```python
from build123d import *

# Parameters (mm, degrees)
EXTRUDE_268_DEPTH      = 3
SKETCH_2_W             = 50
SKETCH_2_H             = 30
CUT_EXTRUDE_486_DEPTH  = 121.867696263
SKETCH_3_R             = 2.5
CUT_EXTRUDE_744_DEPTH  = 121.867696263
SKETCH_4_R             = 2.6
CUT_EXTRUDE_1056_DEPTH = 121.867696263


with BuildPart() as part:
    # 草图1 → Extrude 268 (new body)
    with BuildSketch(Plane(origin=(0, 0, 0), x_dir=(1, 0, 0), z_dir=(0, 1, 0))):
        with BuildLine():
            Line((-100, 50), (100, 50))
            ThreePointArc((100, 50), (107.071067812, 47.071067812), (110, 40))
            Line((110, 40), (110, -40))
            ThreePointArc((110, -40), (107.071067812, -47.071067812), (100, -50))
            Line((100, -50), (-100, -50))
            ThreePointArc((-100, -50), (-107.071067812, -47.071067812), (-110, -40))
            Line((-110, -40), (-110, 40))
            ThreePointArc((-110, 40), (-107.071067812, 47.071067812), (-100, 50))
        make_face()
    extrude(amount=EXTRUDE_268_DEPTH)

    # 草图2 → Cut-Extrude 486 (cut, through all)
    with BuildSketch(Plane(origin=(0, 3, 0), x_dir=(1, 0, 0), z_dir=(0, 1, 0))):
        with Locations((0, 35)):
            Rectangle(SKETCH_2_W, SKETCH_2_H)
    extrude(amount=-CUT_EXTRUDE_486_DEPTH, mode=Mode.SUBTRACT)

    # 草图3 → Cut-Extrude 744 (cut, through all)
    with BuildSketch(Plane(origin=(0, 3, 0), x_dir=(1, 0, 0), z_dir=(0, 1, 0))):
        with Locations(Location((10, 8, 0), (0, 0, 270))):
            Circle(SKETCH_3_R)
        with Locations(Location((10, -12, 0), (0, 0, 270))):
            Circle(SKETCH_3_R)
        with Locations(Location((10, -32, 0), (0, 0, 270))):
            Circle(SKETCH_3_R)
        with Locations(Location((-10, -32, 0), (0, 0, 270))):
            Circle(SKETCH_3_R)
        with Locations(Location((-10, -12, 0), (0, 0, 270))):
            Circle(SKETCH_3_R)
        with Locations(Location((-10, 8, 0), (0, 0, 270))):
            Circle(SKETCH_3_R)
    extrude(amount=-CUT_EXTRUDE_744_DEPTH, mode=Mode.SUBTRACT)

    # 草图4 → Cut-Extrude 1056 (cut, through all)
    with BuildSketch(Plane(origin=(0, 3, 0), x_dir=(1, 0, 0), z_dir=(0, 1, 0))):
        with Locations(Location((100, -35, 0), (0, 0, 270))):
            Circle(SKETCH_4_R)
        with Locations(Location((80, -35, 0), (0, 0, 270))):
            Circle(SKETCH_4_R)
        with Locations(Location((100, -5, 0), (0, 0, 270))):
            Circle(SKETCH_4_R)
        with Locations(Location((80, -5, 0), (0, 0, 270))):
            Circle(SKETCH_4_R)
        with Locations(Location((-100, -35, 0), (0, 0, 270))):
            Circle(SKETCH_4_R)
        with Locations(Location((-100, -5, 0), (0, 0, 270))):
            Circle(SKETCH_4_R)
        with Locations(Location((-80, -35, 0), (0, 0, 270))):
            Circle(SKETCH_4_R)
        with Locations(Location((-80, -5, 0), (0, 0, 270))):
            Circle(SKETCH_4_R)
    extrude(amount=-CUT_EXTRUDE_1056_DEPTH, mode=Mode.SUBTRACT)


solid = part.part
```
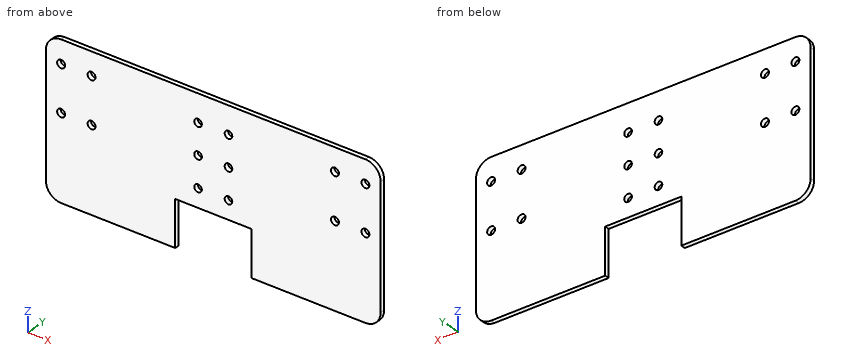
Verification items for the finished model (mm, model axes). Coordinates: 2 decimals unless noted, no trailing zeros. Order: outer loops, then holes, each group sorted by start corner. A loop starts at its lowest first (then second) coordinate and runs counter-clockwise, first axis right, second up. Notation, with made-up numbers: (47.5, 78) -> (58.5, 78) arc R18 ccw to (58.5, 101) -> close; hole circle Ø10 at (18, -3.5). An arc over 180 degrees is marked (long way). Put each result on its own line as item: value. Start each with the question number.
1) Cross-section at A-A (z = 12). Enter the section's corners in (x, y), plus the area to 3 significant figures.
2) Cross-section at B-B (y = 0.65). State how many separate pieces and enclosed holes the cut face has, plus the area to 3 significant figures.
3) Material ranges on L1, parallel to X at y = 1.65, z = 12; L2, parallel to X at y = 1.1, z = 35; L3, parallel to Z at x = 8.5, y = 2, recorded low to high.
4) Cross-section at C-C (x = -80). Enter the section's corners in (y, z), plus the area to 3 significant figures.
5) Cross-section at D-D (x = 10). Enter the section's corners in (y, z), plus the area to 3 significant figures.
Geometry check:
1. outline: (-110, 0) -> (-12.5, 0) -> (-12.5, 3) -> (-110, 3) -> close; (-7.5, 0) -> (7.5, 0) -> (7.5, 3) -> (-7.5, 3) -> close; (12.5, 0) -> (110, 0) -> (110, 3) -> (12.5, 3) -> close
1. area: 630 mm^2
2. separate pieces: 1
2. enclosed holes: 14
2. area: 20,100 mm^2
3. L1: x = -110 to -12.5, -7.5 to 7.5, 12.5 to 110
3. L2: x = -110 to -102.6, -97.4 to -82.6, -77.4 to 77.4, 82.6 to 97.4, 102.6 to 110
3. L3: z = -20 to -10, -6 to 10, 14 to 30, 34 to 50
4. outline: (0, -50) -> (3, -50) -> (3, 2.4) -> (0, 2.4) -> close; (0, 7.6) -> (3, 7.6) -> (3, 32.4) -> (0, 32.4) -> close; (0, 37.6) -> (3, 37.6) -> (3, 50) -> (0, 50) -> close
4. area: 269 mm^2
5. outline: (0, -20) -> (3, -20) -> (3, -10.5) -> (0, -10.5) -> close; (0, -5.5) -> (3, -5.5) -> (3, 9.5) -> (0, 9.5) -> close; (0, 14.5) -> (3, 14.5) -> (3, 29.5) -> (0, 29.5) -> close; (0, 34.5) -> (3, 34.5) -> (3, 50) -> (0, 50) -> close
5. area: 165 mm^2
